from build123d import *

# Parameters (mm, degrees)
SKETCH_3_W               = 180
SKETCH_3_H               = 180
EXTRUDE_1_DEPTH          = 70
SKETCH_5_OUTSIDE_W       = 234.802
SKETCH_5_OUTSIDE_H       = 234.802
SKETCH_5_OUTSIDE_W_2     = 160
SKETCH_5_OUTSIDE_H_2     = 160
CUT_EXTRUDE_1_DEPTH      = 10
SKETCH_6_W               = 13
SKETCH_6_H               = 10
CUT_EXTRUDE_2_DEPTH      = 53
CUT_EXTRUDE_3_REACH      = 147.258
SKETCH_7_R               = 2.5
SKETCH_8_R               = 4
CUT_EXTRUDE_4_DEPTH      = 2
SKETCH_9_R               = 33.5
EXTRUDE_2_DEPTH          = 38
SKETCH_10_R              = 12
EXTRUDE_3_DEPTH          = 16.4
SKETCH_11_W              = 44
SKETCH_11_H              = 22
CUT_EXTRUDE_5_DEPTH      = 3
PATTERN_CIRCULAR_1_COUNT = 3
CUT_EXTRUDE_6_REACH      = 147.258
SKETCH_12_W              = 13
SKETCH_12_H              = 7
PATTERN_CIRCULAR_2_COUNT = 3
SKETCH_13_W              = 160
SKETCH_13_H              = 155
CUT_EXTRUDE_7_DEPTH      = 50
CUT_EXTRUDE_START        = -10
CUT_EXTRUDE_8_DEPTH      = 10
SKETCH_20_W              = 43.47623614
SKETCH_20_H              = 54.53887657
EXTRUDE_4_DEPTH          = 28
SWEEP_START              = -15
SWEEP_2_DEPTH            = 30


# Read off the part's stored shape, not the designer's step: 切除-扫描2
with BuildPart() as part:
    # 草图3 → 凸台-拉伸1 (new body)
    with BuildSketch(Plane(origin=(0, 0, 0), x_dir=(1, 0, 0), z_dir=(0, 1, 0))):
        Rectangle(SKETCH_3_W, SKETCH_3_H)
    extrude(amount=EXTRUDE_1_DEPTH)

    # 草图5 outside → 切除-拉伸1 (cut)
    with BuildSketch(Plane(origin=(0, 70, 0), x_dir=(1, 0, 0), z_dir=(0, 1, 0))):
        Rectangle(SKETCH_5_OUTSIDE_W, SKETCH_5_OUTSIDE_H)
        Rectangle(SKETCH_5_OUTSIDE_W_2, SKETCH_5_OUTSIDE_H_2, mode=Mode.SUBTRACT)
    extrude(amount=-CUT_EXTRUDE_1_DEPTH, mode=Mode.SUBTRACT)

    # 草图6 → 切除-拉伸2 (cut)
    with BuildSketch(Plane(origin=(0, 60, 0), x_dir=(1, 0, 0), z_dir=(0, 1, 0))):
        with Locations((0, -85)):
            Rectangle(SKETCH_6_W, SKETCH_6_H)
    extrude(amount=-CUT_EXTRUDE_2_DEPTH, mode=Mode.SUBTRACT)

    # 草图7 → 切除-拉伸3 (cut, up to next)
    with BuildSketch(Plane.XZ, mode=Mode.PRIVATE) as cut_extrude_3_sk1:
        with Locations(Location((0, 85.3, 0), (0, 0, 270))):
            Circle(SKETCH_7_R)
    cut_extrude_3_tool1 = extrude(cut_extrude_3_sk1.sketch, amount=-CUT_EXTRUDE_3_REACH, mode=Mode.PRIVATE) & part.part
    add(cut_extrude_3_tool1.solids().sort_by_distance((0, 0, 85.3))[0], mode=Mode.SUBTRACT)

    # 草图8 → 切除-拉伸4 (cut)
    with BuildSketch(Plane.XZ):
        with Locations(Location((0, 85.3, 0), (0, 0, 270))):
            Circle(SKETCH_8_R)
    extrude(amount=-CUT_EXTRUDE_4_DEPTH, mode=Mode.SUBTRACT)

    # 草图9 → 凸台-拉伸2 (add)
    with BuildSketch(Plane(origin=(0, 70, 0), x_dir=(1, 0, 0), z_dir=(0, 1, 0))):
        with Locations(Location((0, 0, 0), (0, 0, 270))):
            Circle(SKETCH_9_R)
    extrude(amount=EXTRUDE_2_DEPTH)

    # 草图10 → 凸台-拉伸3 (add)
    with BuildSketch(Plane(origin=(0, 108, 0), x_dir=(1, 0, 0), z_dir=(0, 1, 0))):
        with Locations(Location((0, 0, 0), (0, 0, 270))):
            Circle(SKETCH_10_R)
    extrude(amount=EXTRUDE_3_DEPTH)

    # 草图11 → 切除-拉伸5 (cut)
    with BuildSketch(Plane(origin=(0, 70, 0), x_dir=(1, 0, 0), z_dir=(0, 1, 0))):
        with Locations((0, 68)):
            Rectangle(SKETCH_11_W, SKETCH_11_H)
    cut_extrude_5 = extrude(amount=-CUT_EXTRUDE_5_DEPTH, mode=Mode.SUBTRACT)

    # 阵列(圆周)1: 切除-拉伸5 ×3 about axis
    pattern_circular_1_axis = Axis((0, 0, 0), (0, 1, 0))
    for i in range(1, PATTERN_CIRCULAR_1_COUNT):
        add(cut_extrude_5.rotate(pattern_circular_1_axis, i * 360 / PATTERN_CIRCULAR_1_COUNT), mode=Mode.SUBTRACT)

    # 草图12 → 切除-拉伸6 (cut, up to next)
    with BuildSketch(Plane(origin=(0, 70, 0), x_dir=(1, 0, 0), z_dir=(0, 1, 0)), mode=Mode.PRIVATE) as cut_extrude_6_sk1:
        with Locations((0, 53.5)):
            Rectangle(SKETCH_12_W, SKETCH_12_H)
    cut_extrude_6_tool1 = extrude(cut_extrude_6_sk1.sketch, amount=-CUT_EXTRUDE_6_REACH, mode=Mode.PRIVATE) & part.part
    cut_extrude_6 = cut_extrude_6_tool1.solids().sort_by_distance((0, 70, -53.5))[0]
    add(cut_extrude_6, mode=Mode.SUBTRACT)

    # 阵列(圆周)2: 切除-拉伸6 ×3 about axis
    pattern_circular_2_axis = Axis((0, 0, 0), (0, 1, 0))
    for i in range(1, PATTERN_CIRCULAR_2_COUNT):
        add(cut_extrude_6.rotate(pattern_circular_2_axis, i * 360 / PATTERN_CIRCULAR_2_COUNT), mode=Mode.SUBTRACT)

    # 草图13 → 切除-拉伸7 (cut)
    with BuildSketch(Plane.XZ):
        with Locations((0, -2.5)):
            Rectangle(SKETCH_13_W, SKETCH_13_H)
    extrude(amount=-CUT_EXTRUDE_7_DEPTH, mode=Mode.SUBTRACT)

    # 草图14 → 切除-拉伸8 (cut)
    with BuildSketch(Plane(origin=(0, 108, 0), x_dir=(1, 0, 0), z_dir=(0, 1, 0)).offset(CUT_EXTRUDE_START)):
        with BuildLine():
            Line((-8.059494125, -12.650871687), (-17.99953688, -28.253613435))
            ThreePointArc((-17.99953688, -28.253613435), (0, -33.5), (17.99953688, -28.253613435))
            Line((17.99953688, -28.253613435), (8.059494125, -12.650871687))
            ThreePointArc((8.059494125, -12.650871687), (0, -15), (-8.059494125, -12.650871687))
        make_face()
    extrude(amount=CUT_EXTRUDE_8_DEPTH, mode=Mode.SUBTRACT)

    # 草图20 → 凸台-拉伸4 (add)
    with BuildSketch(Plane(origin=(0, 70, 0), x_dir=(1, 0, 0), z_dir=(0, 1, 0))):
        with Locations((-0.01436765, -52.730561715)):
            Rectangle(SKETCH_20_W, SKETCH_20_H)
    extrude(amount=EXTRUDE_4_DEPTH)

    # 切除-扫描2 outline → 切除-扫描2 (cut)
    with BuildSketch(Plane.YZ.offset(SWEEP_START)):
        Polygon((98, 6.738189634), (98, 41.43061062), (75.764947914, 80), (60, 80), (60, 90), (50, 90), align=None)
    extrude(amount=SWEEP_2_DEPTH, mode=Mode.SUBTRACT)


solid = part.part
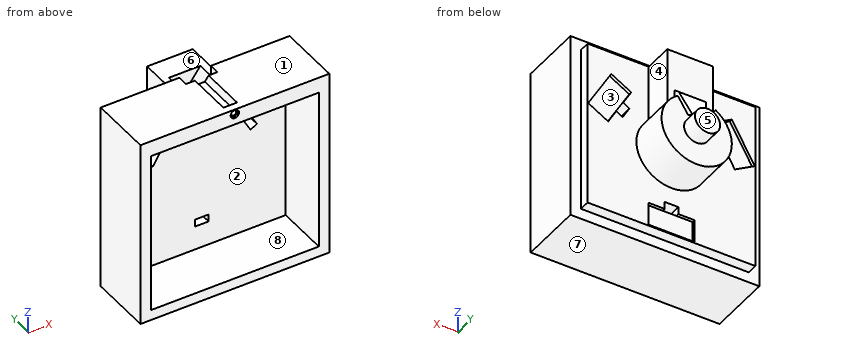
Input: part model. Units: mm. Frame: model coordinates. Face numbers are marked on the shaded views. A direction names the side the tool comes from. Give positions to 0.01 mm unless a question says otherwise; leave off trailing zeros. Loops run counter-clockwise (first coordinate to the right, second up) from the corner with the lowest first, then second, coordinate; pieces in that order, holes last. Notation, with made-up numbers: (82, 54.25) -> (112, 54.25) arc R10 cw to (112, 61.25) -> close; hole circle Ø9 at (36, 68). An arc over 180 degrees is marked (long way). Answer as a JSON object with one key per item and string values. Group by question number.
Item 1: Cut plane B-B, the plane y = 10. Return the cut outline in (x, z), and give its area (3 significant figures).
Item 2: Pin query (flat end, axial travel): P1, Ø8, axis at y = 63.5, z = -37.5, coming from the -X side; P2, Ø6.5, axis at x = 0, z = 85.3, coming from the +Y side; P3, Ø8, axis at y = 66.5, z = -39, coming from the +X side; P4, Ø2.5, axis at y = 68, z = -66.5, coming from the -X side. Return the tip coordinate at first contact, or that it passes through.
Item 3: Cut plane D-D, the plane x = 75. Return the cut outline in (y, z).
Item 4: Line query: probe 1 along Z at (x, y) = (68, 15); probe 2 along X at (y, z) = (17.5, -47); probe 3 along X at (y, z) = (0.65, 85.3). Output: solid intervals per line, ascending.
Item 5: Pull-direction query (Z, two-part tool) for the marked faces 6, 7 and 8; classes: released by +Z, released by -Z, zero draft, split by the parting line, or undercut.
Item 6: Reachability of the marked faces 1, 2, 3, 4 and 5 from +Z, -Z, +X, -X, +Y, -Y: full face, straight path, thin tool, end or side. Return the list, or none.
Item 7: Cut plane C-C, the plane z = 85.3. Return the cut outline in (x, y), and give its area (3 significant figures).
Item 8: Cut plane A-A, the plane z = -65.5. Return the cut outline in (x, y), and give its area (3 significant figures).
Checks:
{
 "1": {"outline": "(-90, -90) -> (90, -90) -> (90, 90) -> (6.5, 90) -> (6.5, 80) -> (-6.5, 80) -> (-6.5, 90) -> (-90, 90) -> close; hole (-80, -80) -> (80, -80) -> (80, 75) -> (-80, 75) -> close", "area": "7,470 mm²"},
 "2": {"P1": "stops at x = -90", "P2": "stops at y = 7", "P3": "stops at x = 80", "P4": "stops at x = -80"},
 "3": {"outline": "(0, -90) -> (60, -90) -> (60, -80) -> (70, -80) -> (70, 17.9) -> (67, 17.9) -> (67, 28.1) -> (70, 28.1) -> (70, 80) -> (60, 80) -> (60, 90) -> (0, 90) -> (0, 75) -> (50, 75) -> (50, -80) -> (0, -80) -> close"},
 "4": {"probe 1": "z = -90 to -80, 75 to 90", "probe 2": "x = -90 to -80, 80 to 90", "probe 3": "x = -90 to -4, 4 to 90"},
 "5": {"face 6": "released by +Z", "face 7": "released by -Z", "face 8": "undercut"},
 "6": {"face 1": "+Z, +X, -X, +Y, -Y", "face 2": "-Y", "face 3": "+Y", "face 4": "+Z, +X, +Y", "face 5": "+Z, -Z, +X, -X, +Y"},
 "7": {"outline": "(-90, 0) -> (-4, 0) -> (-4, 2) -> (-2.5, 2) -> (-2.5, 7) -> (-6.5, 7) -> (-6.5, 52.71) -> (-15, 52.71) -> (-15, 60) -> (-90, 60) -> close; (2.5, 2) -> (4, 2) -> (4, 0) -> (90, 0) -> (90, 60) -> (15, 60) -> (15, 52.71) -> (6.5, 52.71) -> (6.5, 7) -> (2.5, 7) -> close", "area": "9,950 mm²"},
 "8": {"outline": "(-90, 0) -> (-80, 0) -> (-80, 50) -> (80, 50) -> (80, 0) -> (90, 0) -> (90, 60) -> (80, 60) -> (80, 70) -> (22, 70) -> (22, 67) -> (-22, 67) -> (-22, 70) -> (-80, 70) -> (-80, 60) -> (-90, 60) -> close", "area": "4,270 mm²"}
}
